from build123d import *

# Parameters (mm, degrees)
SKETCH1_R               = 44
BOSS_EXTRUDE1_DEPTH     = 130
SKETCH2_R               = 39.5
CUT_EXTRUDE1_DEPTH      = 90
SKETCH3_R               = 39.5
CUT_EXTRUDE2_DEPTH      = 35
SKETCH6_W               = 11.193141888
SKETCH6_H               = 132.356748066
CUT_EXTRUDE3_DEPTH      = 95
SKETCH7_W               = 11.193141888
SKETCH7_H               = 11.193141887
CUT_EXTRUDE4_DEPTH      = 25
CUT_EXTRUDE5_DEPTH      = 5
SKETCH11_W              = 10
SKETCH11_H              = 10
CUT_EXTRUDE6_DEPTH      = 5
CUT_EXTRUDE6_DEPTH_BACK = 5


with BuildPart() as part:
    # Sketch1 → Boss-Extrude1 (new body)
    with BuildSketch(Plane.XY):
        Circle(SKETCH1_R)
    extrude(amount=BOSS_EXTRUDE1_DEPTH)

    # Sketch2 → Cut-Extrude1 (cut)
    with BuildSketch(Plane(origin=(0, 0, 0), x_dir=(-1, 0, 0), z_dir=(0, 0, -1))):
        Circle(SKETCH2_R)
    extrude(amount=-CUT_EXTRUDE1_DEPTH, mode=Mode.SUBTRACT)

    # Sketch3 → Cut-Extrude2 (cut)
    with BuildSketch(Plane.XY.offset(130)):
        Circle(SKETCH3_R)
    extrude(amount=-CUT_EXTRUDE2_DEPTH, mode=Mode.SUBTRACT)

    # Sketch6 → Cut-Extrude3 (cut)
    with BuildSketch(Plane(origin=(0, 42, 0), x_dir=(1, 0, 0), z_dir=(0, 1, 0))):
        with Locations((0, -58)):
            Rectangle(SKETCH6_W, SKETCH6_H)
    extrude(amount=CUT_EXTRUDE3_DEPTH, mode=Mode.SUBTRACT)

    # Sketch7 → Cut-Extrude4 (cut)
    with BuildSketch(Plane(origin=(0, 42, 0), x_dir=(1, 0, 0), z_dir=(0, 1, 0))):
        with Locations((0, -118.581803089)):
            Rectangle(SKETCH7_W, SKETCH7_H)
    extrude(amount=-CUT_EXTRUDE4_DEPTH, mode=Mode.SUBTRACT)

    # Sketch9 → Cut-Extrude5 (cut)
    with BuildSketch(Plane(origin=(0, 0, 0), x_dir=(-1, 0, 0), z_dir=(0, 0, -1))):
        with BuildLine():
            Line((14.535856091, 39.936936383), (13.851815805, 38.057551142))
            ThreePointArc((13.851815805, 38.057551142), (0, -40.5), (-13.851815805, 38.057551142))
            Line((-13.851815805, 38.057551142), (-14.535856091, 39.936936383))
            ThreePointArc((-14.535856091, 39.936936383), (0, -42.5), (14.535856091, 39.936936383))
        make_face()
    cut_extrude5 = extrude(amount=-CUT_EXTRUDE5_DEPTH, mode=Mode.SUBTRACT)

    # Sketch11 → Cut-Extrude6 (cut, two sides)
    with BuildSketch(Plane(origin=(40, 0, 0), x_dir=(0, 0, -1), z_dir=(1, 0, 0))) as cut_extrude6_sk:
        with Locations((-119.2, 0)):
            Rectangle(SKETCH11_W, SKETCH11_H)
    extrude(amount=CUT_EXTRUDE6_DEPTH, mode=Mode.SUBTRACT)
    extrude(cut_extrude6_sk.sketch, amount=-CUT_EXTRUDE6_DEPTH_BACK, mode=Mode.SUBTRACT)

    # Mirror1: Cut-Extrude5 across plane
    add(cut_extrude5.mirror(Plane(origin=(0, 0, 65), x_dir=(1, 0, 0), z_dir=(0, 0, -1))), mode=Mode.SUBTRACT)


solid = part.part
Build history of the part. All positions in model axes, mm. A direction names the side the tool comes from. Give positions to 0.01 mm unless a question says otherwise; leave off trailing zeros. Write each loop counter-clockwise with the first axis right and the second up, starting at its lowest first coordinate (ties: lowest second). Pieces come first, ordered by that corner, then holes. Notation, with made-up numbers: (37.5, 19.5) - (62.5, 19.5) arc R22 ccw to (62.5, 52.5) - close; hole circle Ø1 at (77.5, 40.25). An arc over 180 degrees is marked (long way). Use one line per item in the form item = value. Start each with the question number.
1. 3-axis set-ups, long thin cutter, end or side, ignore diameter. For faces 1 (the face through (0, 42, 124.178)), 2 (the face through (-1.58, -40.47, 127.54)), 3 (the face through (41, 5, 119)): which of +Z, -Z, +X, -X, +Y, -Y reach the whole face in a straight line?
2. Probe line 1 (Y direction, x = 0, z = 1.75); line 2 (Y direction, x = 0, z = 57.5); line 3 (Z direction, x = 34.5, y = 19). List the from-to ranges inside material, lowest first. Write a range as [from, to].
3. Band-saw the part on D-D on y = -35.5. Write the cut outline in (x, z).
4. Two-plate mould, pull along X, no slides. Class faces 4 (the face through (-9.538, -42.954, 64.09)), 5 (the face through (-39.3, 6.5, 0)), 6 (the face through (-1, 1, 95)): released by +X, released by -X, zero draft, split by the parting line, or undercut.
5. Band-saw the part on B-B on x = 0. Write the cut outline in (y, z), plus the area to 3 significant figures.
6. Band-saw the part on C-C on z = 59.5. Write the cut outline in (x, y).
7. Drop flat-ended pins along their axis: pin 1 Ø1 at (x, z) = (33, 61.5) entering from +Y; pin 2 Ø5.5 at (x, z) = (-1.5, 57) entering from +Y; pin 3 Ø2.5 at (y, z) = (41, 53.5) entering from -X. Give the stop position or say it passes through.
Conclusion:
q1.face_1 = +Y
q1.face_2 = +Z
q1.face_3 = +X
q2.line_1 = [-44, -42.5], [-40.5, -39.5], [39.5, 42]
q2.line_2 = [-44, -39.5], [39.5, 42]
q2.line_3 = [90, 95]
q3.outline = (-26, 0) - (-23.37, 0) - (-23.37, 5) - (-19.49, 5) - (-19.49, 0) - (-17.32, 0) - (-17.32, 90) - (17.32, 90) - (17.32, 0) - (19.49, 0) - (19.49, 5) - (23.37, 5) - (23.37, 0) - (26, 0) - (26, 130) - (23.37, 130) - (23.37, 125) - (19.49, 125) - (19.49, 130) - (17.32, 130) - (17.32, 95) - (-17.32, 95) - (-17.32, 130) - (-19.49, 130) - (-19.49, 125) - (-23.37, 125) - (-23.37, 130) - (-26, 130) - close
q4.face_4 = split by the parting line
q4.face_5 = zero draft
q4.face_6 = undercut
q5.outline = (-44, 0) - (-42.5, 0) - (-42.5, 5) - (-40.5, 5) - (-40.5, 0) - (-39.5, 0) - (-39.5, 90) - (39.5, 90) - (39.5, 0) - (42, 0) - (42, 112.99) - (39.5, 112.99) - (39.5, 95) - (-39.5, 95) - (-39.5, 130) - (-40.5, 130) - (-40.5, 125) - (-42.5, 125) - (-42.5, 130) - (-44, 130) - close; (39.5, 124.18) - (44, 124.18) - (44, 130) - (39.5, 130) - close
q5.area = 1,270 mm²
q6.outline = (-5.6, 42) - (-5.6, 43.64) arc R44 ccw (long way) to (5.6, 43.64) - (5.6, 42) - close; hole circle Ø79 at (0, 0)
q7.pin_1 = 29.66
q7.pin_2 = 42
q7.pin_3 = -18.87
